Part model, mm, in its own coordinate system. A direction names the side the tool comes from. Give positions to 0.01 mm unless a question says otherwise; leave off trailing zeros.
```python
from build123d import *

# Parameters (mm, degrees)
F1_ANGLE  = 180
F3_ANGLE  = 180
F5_R      = 1.5875
F6_DEPTH  = 3.175
F7_R      = 1.9685
F8_DEPTH  = 6.858
F10_ANGLE = 180


with BuildPart() as f1:
    # F0 (on Front) → F1 (revolve)
    with BuildSketch(Plane.XZ):
        Polygon((82.296, 0), (76.2, 0), (76.2, -5.08), (78.486, -5.08), (78.486, -10.922), (79.756, -10.922), (79.756, -5.08), (82.296, -5.08), align=None)
    revolve(axis=Axis((0, 0, -3.3090594225), (0, 0, -1)), revolution_arc=F1_ANGLE)

    # F2 (on face) → F3 (revolve)
    with BuildSketch(Plane(origin=(0, 0, 0), x_dir=(-1, 0, 0), z_dir=(0, 1, 0))):
        with BuildLine():
            Line((109.982, 107.95), (107.95, 107.95))
            Line((107.95, 107.95), (107.95, 95.4419970512))
            Line((107.95, 95.4419970512), (109.9555790424, 86.0509946942))
            add(Edge.make_bspline(
                [(109.9555790424, 86.0509946942), (110.2117663194, 83.2401192533), (110.6106504967, 76.722351273), (105.9962332065, 57.8653367135), (101.756604934, 45.6968411425), (94.8213054674, 35.4374632093), (89.3245305774, 25.0347896967), (81.0594552677, 8.2140825247), (77.5917934991, 2.3874851052), (76.2, 0)],
                knots=[0, 0, 0, 0, 0.119269968, 0.291866141, 0.4362120888, 0.5707580275, 0.708802049, 0.8790644733, 1, 1, 1, 1], degree=3))
            Line((76.2, 0), (82.296, 0))
            add(Edge.make_bspline(
                [(82.296, 0), (83.3510677988, 2.7460559383), (86.9251299009, 8.3371760807), (92.2485769181, 22.0550745253), (104.7864032306, 41.4168156388), (113.5254737482, 65.4432313512), (117.0270400805, 95.0726980879), (114.3, 107.95)],
                knots=[0, 0, 0, 0, 0.1305115226, 0.2947178963, 0.4990111446, 0.7205265486, 1, 1, 1, 1], degree=3))
            Line((114.3, 107.95), (111.76, 107.95))
            Line((111.76, 107.95), (111.76, 100.7509976625))
            Line((111.76, 100.7509976625), (109.982, 100.7509976625))
            Line((109.982, 100.7509976625), (109.982, 107.95))
        make_face()
    revolve(axis=Axis((0, 0, 53.975), (0, 0, 1)), revolution_arc=F3_ANGLE)

    # F5 (on face) → F6 (join)
    with BuildSketch(Plane(origin=(0, 0, 0), x_dir=(-1, 0, 0), z_dir=(0, 1, 0))):
        with Locations((111.76, 95.25)):
            Circle(F5_R)
        with Locations((79.4557631016, 0)):
            Circle(F5_R)
        with Locations((109.0777590871, 62.0304606855)):
            Circle(F5_R)
        with Locations((-111.76, 95.25)):
            Circle(F5_R)
        with Locations((-109.0777590871, 62.0304606855)):
            Circle(F5_R)
        with Locations((-79.4557631016, 0)):
            Circle(F5_R)
    extrude(amount=F6_DEPTH)

    # F7 (on face) → F8 (cut)
    with BuildSketch(Plane(origin=(0, 3.175, 0), x_dir=(-1, 0, 0), z_dir=(0, 1, 0))):
        with Locations((-111.76, 95.25)):
            Circle(F7_R)
        with Locations((-109.0668961406, 62.0584301651)):
            Circle(F7_R)
        with Locations((-79.4181898236, 0)):
            Circle(F7_R)
    extrude(amount=-F8_DEPTH, mode=Mode.SUBTRACT)

    # F9 (on face) → F10 (revolve)
    with BuildSketch(Plane(origin=(0, 0, 0), x_dir=(-1, 0, 0), z_dir=(0, 1, 0))):
        Polygon((-81.896, -5.08), (-82.296, -5.08), (-82.296, -10.922), (-81.096, -10.922), (-81.096, -5.7301754132), align=None)
        Polygon((-76.2, -10.922), (-76.2, -5.08), (-76.6, -5.08), (-77.4, -5.6824819185), (-77.4, -10.922), align=None)
    revolve(axis=Axis((0, 0, -7.6545081101), (0, 0, -1)), revolution_arc=F10_ANGLE)


solid = f1.part
```
1) Wall check: L1, parallel to X at y = -2, z = 95; L2, parallel to X at y = -69, z = 85; L3, parallel to X at y = -4, z = 49. Give the ranges that are in metal, low to high.
Answers follow:
L1: x = -115.59 to -108.03, 108.03 to 109.81, 113.71 to 115.59
L2: x = -92.28 to -85.73, 85.73 to 92.28
L3: x = -107.12 to -102.61, 102.61 to 107.12
2) 3-axis set-ups, long thin cutter, end or side, ignore diameter. For faces 1 (the face through (6.3, -78.5, -10.922)), 2 (the face through (1.7, -77.38, -8.34)), 3 (the face through (9, -110, 100.751)), 4 (the face through (1.786, -81.215, -5.617)), 5 (the face through (1.68, -76.18, -5.54)): which of +Z, -Z, +X, -X, +Y, -Y reach the whole face in a straight line?
Answers follow:
face 1: -Z, +X, -X, +Y, -Y
face 2: -Z
face 3: +Z
face 4: none
face 5: +Z, -Z, +Y
3) Pin check, flat tips, straight feed: pin 1 Ø4 at (x, y) = (51, -52.5) entering from -Z; pin 2 Ø3 at (x, z) = (109.07, 62.06) entering from +Y; pin 3 Ø12 at (x, z) = (-98, 38.5) entering from +Y; pin 4 Ø1 at (y, z) = (-58.5, 64.5) entering from +X. Stop position of each tip, or through.
Answers follow:
pin 1: passes through
pin 2: stops at y = -3.68
pin 3: stops at y = 0
pin 4: stops at x = 95.79
4) Two-plate mould, pull along Z, no slides. Class faces 6 (the face through (-2.418, -109.955, 104.401)), 7 (the face through (0, -77, -5.08)), 8 (the face through (-6.5, -81, -10.922)): +Z half, -Z half, draft (parallel to the pull), parting line (faces both ways), or undercut.
Answers follow:
face 6: draft
face 7: undercut
face 8: -Z half
